from build123d import *

# Parameters (mm, degrees)
EXTRUDE_1_DEPTH     = 37
EXTRUDE_1_2_DEPTH   = 37
SKETCH_1_4_R        = 20
SKETCH_1_4_W        = 50
SKETCH_1_4_H        = 18.464991829
EXTRUDE_2_DEPTH     = 50
SKETCH_3_R          = 4
CUT_EXTRUDE_1_DEPTH = 54
FILLET_1_R          = 20


with BuildPart() as part:
    # Sketch 1 → Extrude 1 (new body)
    with BuildSketch(Plane.XY):
        with BuildLine():
            Line((-25, 25), (-25, 6.535008171))
            Line((-25, 6.535008171), (-18.902213315, 6.535008171))
            ThreePointArc((-18.902213315, 6.535008171), (0, 20), (18.902213315, 6.535008171))
            Line((18.902213315, 6.535008171), (25, 6.535008171))
            Line((25, 6.535008171), (25, 25))
            Line((25, 25), (-25, 25))
        make_face()
    extrude(amount=EXTRUDE_1_DEPTH)



with BuildPart() as body_2:
    # Sketch 1 → Extrude 1 2 (new body)
    with BuildSketch(Plane.XY):
        with BuildLine():
            Line((-18.902213315, -6.535008171), (-25, -6.535008171))
            Line((-25, -6.535008171), (-25, -25))
            Line((-25, -25), (25, -25))
            Line((25, -25), (25, -6.535008171))
            Line((25, -6.535008171), (18.902213315, -6.535008171))
            ThreePointArc((18.902213315, -6.535008171), (0, -20), (-18.902213315, -6.535008171))
        make_face()
    extrude(amount=EXTRUDE_1_2_DEPTH)


with BuildPart() as part_1:
    add(part.part)

    add(body_2.part)  # Extrude 2 merges body 2
    # Sketch 1_4 → Extrude 2 (add)
    with BuildSketch(Plane.XY):
        Circle(SKETCH_1_4_R)
        with Locations((0, 15.767504086)):
            Rectangle(SKETCH_1_4_W, SKETCH_1_4_H)
        with BuildLine():
            ThreePointArc((18.902213315, 6.535008171), (0, 20), (-18.902213315, 6.535008171))
            Line((-18.902213315, 6.535008171), (18.902213315, 6.535008171))
        make_face()
        with BuildLine():
            Line((18.902213315, 6.535008171), (-18.902213315, 6.535008171))
            ThreePointArc((-18.902213315, 6.535008171), (-20, 0), (-18.902213315, -6.535008171))
            Line((-18.902213315, -6.535008171), (18.902213315, -6.535008171))
            ThreePointArc((18.902213315, -6.535008171), (19.723644013, -3.313286412), (20, 0))
            ThreePointArc((20, 0), (19.723644013, 3.313286412), (18.902213315, 6.535008171))
        make_face()
        with BuildLine():
            Line((-18.902213315, 6.535008171), (-25, 6.535008171))
            Line((-25, 6.535008171), (-25, -6.535008171))
            Line((-25, -6.535008171), (-18.902213315, -6.535008171))
            ThreePointArc((-18.902213315, -6.535008171), (-20, 0), (-18.902213315, 6.535008171))
        make_face()
        with BuildLine():
            Line((25, 6.535008171), (18.902213315, 6.535008171))
            ThreePointArc((18.902213315, 6.535008171), (19.723644013, 3.313286412), (20, 0))
            ThreePointArc((20, 0), (19.723644013, -3.313286412), (18.902213315, -6.535008171))
            Line((18.902213315, -6.535008171), (25, -6.535008171))
            Line((25, -6.535008171), (25, 6.535008171))
        make_face()
        with BuildLine():
            Line((18.902213315, -6.535008171), (-18.902213315, -6.535008171))
            ThreePointArc((-18.902213315, -6.535008171), (0, -20), (18.902213315, -6.535008171))
        make_face()
        with Locations((0, -15.767504086)):
            Rectangle(SKETCH_1_4_W, SKETCH_1_4_H)
    extrude(amount=-EXTRUDE_2_DEPTH)

    # Sketch 3 → Cut-Extrude 1 (cut)
    with BuildSketch(Plane.ZY.offset(25)):
        with Locations((-25, 0)):
            Circle(SKETCH_3_R)
    extrude(amount=-CUT_EXTRUDE_1_DEPTH, mode=Mode.SUBTRACT)

    # Fillet 1
    fillet_1_edges = [part_1.edges().sort_by_distance(p)[0] for p in [
        (0, -25, -50),
        (0, 25, -50),
    ]]
    fillet(fillet_1_edges, radius=FILLET_1_R)


solid = part_1.part
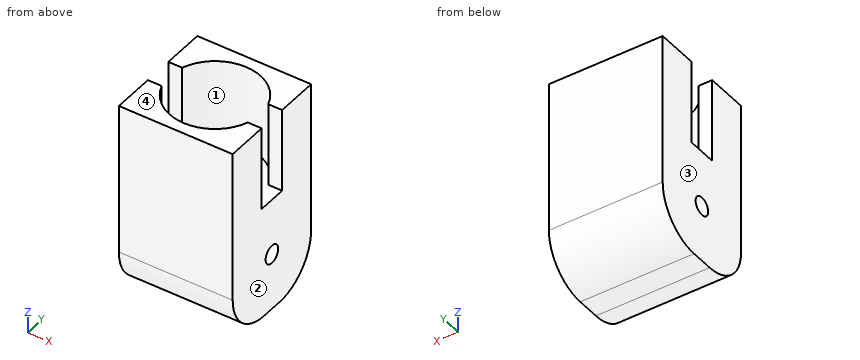
Could you check a few things on this model? Use its own coordinates, in mm. Face numbers are marked on the shaded views. Give positions to 0.01 mm unless a question says otherwise; leave off trailing zeros. Order: outer loops, then holes, each group sorted by start corner. A loop starts at its lowest first (then second) coordinate and runs counter-clockwise, first axis right, second up. Notation, with made-up numbers: M -35.5,72 L 4.5,72 A22 cw 4.5,100 Z; hole C 27,44.25 d3. An arc over 180 degrees is marked long. One line per question, with ' | ' between items.
1. I want a section at C-C (y = 0). List the corners of the cut face in (x, z) for me, and give its area (3 significant figures).
Results:
outline: M -25,-50 L 25,-50 L 25,-29 L -25,-29 Z; M -25,-21 L 25,-21 L 25,0 L -25,0 Z | area: 2,100 mm²
2. I want a section at B-B (x = -16). List the corners of the cut face in (y, z) for me.
Results:
outline: M -25,-30 A20 ccw -5,-50 L 5,-50 A20 ccw 25,-30 L 25,37 L 12,37 L 12,0 L -12,0 L -12,37 L -25,37 Z; hole C 0,-25 d8
3. I want a section at A-A (z = -25). List the corners of the cut face in (x, y) for me.
Results:
outline: M -25,-25 L 25,-25 L 25,-4 L -25,-4 Z; M -25,4 L 25,4 L 25,25 L -25,25 Z
4. I'm going to push flat-ended pins straight in: pin 1 (6 mm diameter, centred on x = -6.5, y = -3, fed in from +Z); pin 2 (7 mm diameter, centred on y = 0, z = -25, fed in from +X); pin 3 (5 mm diameter, centred on x = -18, y = 12, fed in from -Z). Where does each tip first touch, or does it pass through?
Results:
pin 1: z = 0 | pin 2: through | pin 3: z = -49.49
5. I want a section at D-D (y = -11.5). List the corners of the cut face in (x, z) for me.
Results:
outline: M -25,-48.91 L 25,-48.91 L 25,37 L 16.36,37 L 16.36,0 L -16.36,0 L -16.36,37 L -25,37 Z
6. We'd pull the mould along X, two halves only. Please class the marked faces 1, 2, 3 and 4: +X half, -X half, draft (parallel to the pull), parting line (faces both ways), or undercut.
Results:
face 1: undercut | face 2: +X half | face 3: -X half | face 4: draft
7. If I drill on line 1 (Y direction, x = 8, z = -25); line 2 (Z direction, x = -15, y = 3.5); line 3 (Y direction, x = 4.5, z = 8), over which ranges is the centre line in solid material (lowest first)?
Results:
line 1: -25 to -4, 4 to 25 | line 2: -50 to -26.94, -23.06 to 0 | line 3: -25 to -19.49, 19.49 to 25
